Check sheet for the modelled part. Datum: model origin and axes. Units: mm. A direction names the side the tool comes from. Coordinates: 2 decimals unless noted, no trailing zeros. Write each loop counter-clockwise with the first axis right and the second up, starting at its lowest first coordinate (ties: lowest second). Pieces come first, ordered by that corner, then holes. Notation, with made-up numbers: (81.5, -10.5) -> (134.5, -10.5) arc R29 ccw to (134.5, 19.5) -> close; hole circle Ø2 at (-30, 37). An arc over 180 degrees is marked (long way). One line per item, written item: value. Start each with the question number.
1) Scan lines: line 1 along X through (y, z) = (1.15, -27.75); line 2 along X through (y, z) = (1.8, -48.5); line 3 along Z through (x, y) = (-27, 1.4). Record each from-to range of solid material in increasing order. Write a range as [from, to].
2) Set-up check for faces 1 (the cylindrical face through (-28, 0, 41)), 2 (the cylindrical face through (-38.684, 1.014, 41.839)): record each of +Z, -Z, +X, -X, +Y, -Y from which the full face is reachable in a straight line by a thin tool's end or side.
3) Draft check along X on faces 3 (the cylindrical face through (28, 0, 41)), 4 (the cylindrical face through (-39.39, 1.8, -49.68)), 5 (the cylindrical face through (39.39, 1.8, 49.68)). Enter one of: +X half, -X half, draft (parallel to the pull), parting line (faces both ways), or undercut.
4) Gauge pin test, flat ends, axial feed: P1, Ø6, axis at x = -36, z = -44.5, coming from the +Y side; P2, Ø5, axis at x = 37.01, z = 44.02, coming from the +Y side; P3, Ø2, axis at y = 1, z = 20.5, coming from the +X side; P4, Ø2, axis at x = 0, y = 1, coming from the -Z side. Record the tip position at first contact, or that the pin passes through.
5) Sectioned sample at A-A on x = -20. Enter the section's corners in (y, z), plus the area to 3 significant figures.
6) Sectioned sample at C-C on y = -1.1. Give the number of separate pieces and of enclosed holes in the cut face, plus the area to 3 significant figures.
7) Sectioned sample at B-B on z = -27.75. Enter the section's corners in (x, y), plus the area to 3 significant figures.
```python
from build123d import *

# Parameters (mm, degrees)
BOSS_EXTRUDE1_DEPTH     = 2
CHAMFER1_SIZE           = 4
CHAMFER1_SIZE_2         = 1.200057511
SKETCH2_R               = 1.6
CUT_EXTRUDE1_DEPTH      = 76.106590923
SKETCH3_R               = 2.75
CUT_EXTRUDE2_DEPTH      = 2
MIRROR2_COPY_1_SKETCH_R = 1.6
MIRROR2_COPY_1_DEPTH    = 76.106590923
MIRROR2_COPY_2_SKETCH_R = 2.75
MIRROR2_COPY_2_DEPTH    = 2
FILLET1_R               = 1
SKETCH4_R               = 1.25
CUT_EXTRUDE3_DEPTH      = 76.106590923
SKETCH5_R               = 2.5
CUT_EXTRUDE4_DEPTH      = 76.106590923


with BuildPart() as part:
    # Sketch1 → Boss-Extrude1 (new, symmetric)
    with BuildSketch(Plane(origin=(0, 0, 0), x_dir=(1, 0, 0), z_dir=(0, 1, 0))):
        Polygon((-45, -41.45898034), (-35.72949017, -60), (35.72949017, -60), (45, -41.45898034), (45, 41.45898034), (35.72949017, 60), (-35.72949017, 60), (-45, 41.45898034), align=None)
    extrude(amount=BOSS_EXTRUDE1_DEPTH, both=True)

    # Chamfer1
    # the kernel refuses this chamfer: 4, 1.200057511 mm, written as the material it takes off along each edge
    with BuildSketch(Plane(origin=(-31.085729195, 2, -69.28752195), x_dir=(-0.0099009581726386, -0.9999387300150343, -0.004950479086319294), z_dir=(-0.44721359549995754, 0, 0.8944271909999161)), Plane(origin=(49.643760975, 2, -32.17145839), x_dir=(0.009900958172639964, -0.9999387300150343, -0.004950479086319981), z_dir=(-0.4472135954999578, 0, -0.894427190999916)), Plane(origin=(31.085729195, 2, 69.28752195), x_dir=(0.009900958172639964, -0.9999387300150343, 0.004950479086319981), z_dir=(0.4472135954999578, 0, -0.894427190999916)), Plane(origin=(-49.643760975, 2, 32.17145839), x_dir=(-0.009900958172639964, -0.9999387300150343, 0.004950479086319981), z_dir=(0.4472135954999578, 0, 0.894427190999916))) as chamfer1_piece_1:
        Polygon((CHAMFER1_SIZE * 0.999938730015, CHAMFER1_SIZE * 0.0110696077582), (-CHAMFER1_SIZE_2 * 0.0110696077607, CHAMFER1_SIZE_2 * 0.999938730237), (0, 0), align=None)
    extrude(amount=41.497020588, mode=Mode.SUBTRACT)
    with BuildSketch(Plane(origin=(46.113255381, 2, -60), x_dir=(0, -0.9999387300150343, -0.011069607758202806), z_dir=(-1, 0, 0))) as chamfer1_piece_2:
        Polygon((CHAMFER1_SIZE * 0.999938730015, CHAMFER1_SIZE * 0.0110696077582), (-CHAMFER1_SIZE_2 * 0.0110696077607, CHAMFER1_SIZE_2 * 0.999938730237), (0, 0), align=None)
    extrude(amount=92.226510762, mode=Mode.SUBTRACT)
    with BuildSketch(Plane(origin=(45, 2, 51.842745551), x_dir=(0.011069607758202806, -0.9999387300150343, 0), z_dir=(0, 0, -1)), Plane(origin=(-45, 2, -51.842745551), x_dir=(-0.011069607758202806, -0.9999387300150343, 0), z_dir=(0, 0, 1))) as chamfer1_piece_3:
        Polygon((CHAMFER1_SIZE * 0.999938730015, CHAMFER1_SIZE * 0.0110696077582), (-CHAMFER1_SIZE_2 * 0.0110696077607, CHAMFER1_SIZE_2 * 0.999938730237), (0, 0), align=None)
    extrude(amount=103.685491102, mode=Mode.SUBTRACT)
    with BuildSketch(Plane(origin=(-46.113255381, 2, 60), x_dir=(0, 0.12207157319780508, -0.9925213000319), z_dir=(1, 0, 0))) as chamfer1_piece_4:
        Polygon((CHAMFER1_SIZE_2 * 0.992521300252, -CHAMFER1_SIZE_2 * 0.122071573225), (-CHAMFER1_SIZE * 0.122071573198, -CHAMFER1_SIZE * 0.992521300032), (0, 0), align=None)
    extrude(amount=92.226510762, mode=Mode.SUBTRACT)

    # Sketch2 → Cut-Extrude1 (cut, through all)
    with BuildSketch(Plane.XZ.offset(2)):
        with Locations(Location((-37.010643118, 44.021286236, 0), (0, 0, 270))):
            Circle(SKETCH2_R)
    cut_extrude1 = extrude(amount=-CUT_EXTRUDE1_DEPTH, mode=Mode.SUBTRACT)

    # Sketch3 → Cut-Extrude2 (cut)
    with BuildSketch(Plane(origin=(0, 2, 0), x_dir=(1, 0, 0), z_dir=(0, 1, 0))):
        with Locations(Location((-37.010643118, -44.021286236, 0), (0, 0, 270))):
            Circle(SKETCH3_R)
    cut_extrude2 = extrude(amount=-CUT_EXTRUDE2_DEPTH, mode=Mode.SUBTRACT)

    # Mirror1: Cut-Extrude1, Cut-Extrude2 across plane
    add(cut_extrude1.mirror(Plane(origin=(0, 0, 0), x_dir=(0, 0, 1), z_dir=(1, 0, 0))), mode=Mode.SUBTRACT)
    add(cut_extrude2.mirror(Plane(origin=(0, 0, 0), x_dir=(0, 0, 1), z_dir=(1, 0, 0))), mode=Mode.SUBTRACT)

    # Mirror2: Cut-Extrude1, Cut-Extrude2 across plane
    add(cut_extrude1.mirror(Plane.XY), mode=Mode.SUBTRACT)
    add(cut_extrude2.mirror(Plane.XY), mode=Mode.SUBTRACT)

    # Mirror2 copy 1 sketch → Mirror2 copy 1 (cut, through all)
    with BuildSketch(Plane(origin=(0, -2, 0), x_dir=(-1, 0, 0), z_dir=(0, -1, 0))):
        with Locations(Location((-37.010643118, 44.021286236, 0), (0, 0, 270))):
            Circle(MIRROR2_COPY_1_SKETCH_R)
    extrude(amount=-MIRROR2_COPY_1_DEPTH, mode=Mode.SUBTRACT)

    # Mirror2 copy 2 sketch → Mirror2 copy 2 (cut)
    with BuildSketch(Plane(origin=(0, 2, 0), x_dir=(-1, 0, 0), z_dir=(0, 1, 0))):
        with Locations(Location((-37.010643118, -44.021286236, 0), (0, 0, 270))):
            Circle(MIRROR2_COPY_2_SKETCH_R)
    extrude(amount=-MIRROR2_COPY_2_DEPTH, mode=Mode.SUBTRACT)

    # Fillet1
    fillet1_edges = [part.edges().sort_by_distance(p)[0] for p in [
        (-43.799942489, 2, 0),
        (-39.393878164, 2, 49.98781384),
        (0, 2, 58.799942489),
        (39.393878164, 2, 49.98781384),
        (43.799942489, 2, 0),
        (39.393878164, 2, -49.98781384),
        (0, 2, -58.799942489),
        (-39.393878164, 2, -49.98781384),
        (44.399971244, 0, 41.317332765),
        (35.358652005, 0, 59.399971244),
        (44.399971244, 0, -41.317332765),
        (-35.358652005, 0, 59.399971244),
        (35.358652005, 0, -59.399971244),
        (-44.399971244, 0, 41.317332765),
        (-35.358652005, 0, -59.399971244),
        (-44.399971244, 0, -41.317332765),
    ]]
    fillet(fillet1_edges, radius=FILLET1_R)

    # Sketch4 → Cut-Extrude3 (cut, through all)
    with BuildSketch(Plane(origin=(0, 2, 0), x_dir=(1, 0, 0), z_dir=(0, 1, 0))):
        with Locations(Location((-20, 27.75, 0), (0, 0, 270))):
            Circle(SKETCH4_R)
        with Locations(Location((-28, -42.25, 0), (0, 0, 270))):
            Circle(SKETCH4_R)
        with Locations(Location((20, 27.75, 0), (0, 0, 270))):
            Circle(SKETCH4_R)
        with Locations(Location((28, -42.25, 0), (0, 0, 270))):
            Circle(SKETCH4_R)
    extrude(amount=-CUT_EXTRUDE3_DEPTH, mode=Mode.SUBTRACT)

    # Sketch5 → Cut-Extrude4 (cut, through all)
    with BuildSketch(Plane.XZ.offset(2)):
        with Locations(Location((25, -50, 0), (0, 0, 270))):
            Circle(SKETCH5_R)
        with Locations(Location((-25, -50, 0), (0, 0, 270))):
            Circle(SKETCH5_R)
    extrude(amount=-CUT_EXTRUDE4_DEPTH, mode=Mode.SUBTRACT)


solid = part.part
```
Answers:
1. line 1: x = [-44.05, -21.25], [-18.75, 18.75], [21.25, 44.05]
1. line 2: x = [-39.98, -27], [-23, 23], [27, 39.98]
1. line 3: z = [-58.97, -51.5], [-48.5, 41.5], [43, 58.97]
2. face 1: +Y, -Y
2. face 2: +Y
3. face 3: undercut
3. face 4: -X half
3. face 5: +X half
4. P1: stops at y = 2
4. P2: stops at y = 0
4. P3: stops at x = 44.4
4. P4: stops at z = -59.4
5. outline: (-2, -60) -> (1.29, -59.01) arc R1 ccw to (2, -58.06) -> (2, -29) -> (-2, -29) -> close; (-2, -26.5) -> (2, -26.5) -> (2, 58.06) arc R1 ccw to (1.29, 59.01) -> (-2, 60) -> close
5. area: 465 mm2
6. separate pieces: 1
6. enclosed holes: 10
6. area: 10,300 mm2
7. outline: (-45, -2) -> (-21.25, -2) -> (-21.25, 2) -> (-43.06, 2) arc R1 ccw to (-44.01, 1.29) -> close; (-18.75, -2) -> (18.75, -2) -> (18.75, 2) -> (-18.75, 2) -> close; (21.25, -2) -> (45, -2) -> (44.01, 1.29) arc R1 ccw to (43.06, 2) -> (21.25, 2) -> close
7. area: 335 mm2
